```python
from build123d import *

# Parameters (mm, degrees)
SKETCH_1_R               = 20
EXTRUDE_1_DEPTH          = 55
SKETCH_2_W               = 100
SKETCH_2_H               = 110
EXTRUDE_2_DEPTH          = 10
SKETCH_3_R               = 10
CUT_EXTRUDE_1_DEPTH      = 151
CUT_EXTRUDE_3_DEPTH      = 119.004237212
CUT_EXTRUDE_3_DEPTH_BACK = 119.004237212


with BuildPart() as part:
    # 草图1 → 凸台-拉伸1 (new, symmetric)
    with BuildSketch(Plane.XY):
        Circle(SKETCH_1_R)
    extrude(amount=EXTRUDE_1_DEPTH, both=True)

    # 草图2 → 凸台-拉伸2 (add, symmetric)
    with BuildSketch(Plane(origin=(0, 0, 0), x_dir=(1, 0, 0), z_dir=(0, 1, 0))):
        with Locations((-50, 0)):
            Rectangle(SKETCH_2_W, SKETCH_2_H)
    extrude(amount=EXTRUDE_2_DEPTH, both=True)

    # 草图3 → 切除-拉伸1 (cut, through all)
    with BuildSketch(Plane.XY.offset(55)):
        Circle(SKETCH_3_R)
    extrude(amount=-CUT_EXTRUDE_1_DEPTH, mode=Mode.SUBTRACT)

    # 草图5 → 切除-拉伸3 (cut, two sides: drawn at the far end of the back side and taken through both)
    with BuildSketch(Plane(origin=(0, 10, 0), x_dir=(1, 0, 0), z_dir=(0, 1, 0)).offset(-CUT_EXTRUDE_3_DEPTH_BACK)):
        Polygon((20, -40), (-17.320508076, -18.452994616), (-17.320508076, 18.452994616), (20, 40), align=None)
    extrude(amount=CUT_EXTRUDE_3_DEPTH + CUT_EXTRUDE_3_DEPTH_BACK, mode=Mode.SUBTRACT)


solid = part.part
```
For this review, take the finished solid that the model builds, in its own axes (mm). A direction names the side the tool comes from. Round coordinates to 2 decimals unless told otherwise and drop trailing zeros. Loops run counter-clockwise (first coordinate to the right, second up) from the corner with the lowest first, then second, coordinate; pieces in that order, holes last.
Q1. Add section B-B on y = 11.5. Write out the cut boundary in (x, z).
Result sheet:
outline: (-16.36, -55) - (16.36, -55) - (16.36, -37.9) - (-16.36, -19.01) - close; (-16.36, 19.01) - (16.36, 37.9) - (16.36, 55) - (-16.36, 55) - close
Q2. Mouldability with a two-part tool opening along Y and no side actions: class faces 4 (the face through (-59, -10, -1)), 5 (the face through (7.243, -18.642, -40.531)), 6 (the face through (-8, -6, -42)) as +Y half, -Y half, draft (parallel to the pull), parting line (faces both ways), or undercut.
Result sheet:
face 4: -Y half
face 5: parting line
face 6: undercut
Q3. To check wall thickness, follow line 1 along Y through (x, z) = (0, -40); line 2 along X through (y, z) = (0, 44); line 3 along X through (y, z) = (0, 30). State the ranges of each line that lie inside material, in increasing order.
Result sheet:
line 1: y = -20 to -10, 10 to 20
line 2: x = -100 to -10, 10 to 20
line 3: x = -100 to -10
Q4. Add section A-A on x = 0. Write out the cut boundary in (y, z), plus the area to 3 significant figures.
Result sheet:
outline: (-20, -55) - (-10, -55) - (-10, -28.45) - (-20, -28.45) - close; (-20, 28.45) - (-10, 28.45) - (-10, 55) - (-20, 55) - close; (10, -55) - (20, -55) - (20, -28.45) - (10, -28.45) - close; (10, 28.45) - (20, 28.45) - (20, 55) - (10, 55) - close
area: 1,060 mm2
Q5. Insertion check: pin 1 Ø1 at (y, z) = (16, -22.5) entering from +X; pin 2 Ø5 at (x, z) = (-9, -29) entering from +Y; pin 3 Ø5 at (x, z) = (-81, 2.5) entering from +Y; pin 4 Ø23 at (x, y) = (0, 0) entering from -Z. Each pin has a flat end and moves straight along its axis. Give the tip position at first contact, or say it passes through.
Result sheet:
pin 1: stops at x = -9.44
pin 2: stops at y = 18.91
pin 3: stops at y = 10
pin 4: stops at z = -55
Q6. Machinability: for faces 1 (the face through (-17.321, 0, 0)), 2 (the face through (-59, 10, -1)), 3 (the face through (-41, 0, 55)), which of the approach directions +Z, -Z, +X, -X, +Y, -Y give a long, thin tool a straight path to every point of the face, cutting with its end or side? Answer none if there is none.
Result sheet:
face 1: +X, +Y, -Y
face 2: +Z, -Z, -X, +Y
face 3: +Z, +X, -X, +Y, -Y
Q7. Add section D-D on z = -9. Write out the cut boundary in (x, y), plus the area to 3 significant figures.
Result sheet:
outline: (-100, -10) - (-17.32, -10) - (-17.32, 10) - (-100, 10) - close
area: 1,650 mm2
Q8. Add section C-C on y = -7. Write out the cut boundary in (x, z) (1 decimal), plus the area to 3 significant figures.
Result sheet:
outline: (-100, -55) - (-7.1, -55) - (-7.1, -24.3) - (-17.3, -18.5) - (-17.3, 18.5) - (-7.1, 24.3) - (-7.1, 55) - (-100, 55) - close; (7.1, -55) - (18.7, -55) - (18.7, -39.3) - (7.1, -32.6) - close; (7.1, 32.6) - (18.7, 39.3) - (18.7, 55) - (7.1, 55) - close
area: 10,200 mm2
